Can you work these out from the model? Positions are in its coordinate system, mm. Face numbers are marked on the shaded views. A direction names the side the tool comes from. Round coordinates to 2 decimals unless told otherwise and drop trailing zeros. Write each loop counter-clockwise with the first axis right and the second up, starting at its lowest first coordinate (ties: lowest second). Pieces come first, ordered by that corner, then holes. Notation, with made-up numbers: M 15.25,-19.75 L 21.25,-19.75 A17 ccw 21.25,3.25 Z; hole C -36.75,-15 d7. An arc over 180 degrees is marked long. Answer in a Markdown table with one row per item. Add a question column.
(1) Suppose I cut it at B-B, the plane y = -11. Write out the boundary of the cut face in (x, z), then the cut area to 3 significant figures.
(2) If I drill on probe 1 along X at (y, z) = (-17.65, 0); probe 2 along X at (y, z) = (-14, 0.75); probe 3 along X at (y, z) = (-10, 2.5), over which ranges is the centre line in solid material (lowest first)?
(3) I'm going to push flat-ended pins straight in: pin 1 (2 mm diameter, centred on x = 0, z = 0, fed in from +Y); pin 2 (2 mm diameter, centred on x = 0, z = 0, fed in from -Y); pin 3 (2 mm diameter, centred on x = 1.5, y = 3, fed in from -Z). Where does each tip first touch, or does it pass through?
(4) Suppose I cut it at A-A, the plane y = 17. Write out the boundary of the cut face in (x, z), then the cut area to 3 significant figures.
(5) If we mould it in two halves opening along Z, with no side actions, what happens to the marked faces 1, 2 and 3? For each: released by +Z, released by -Z, zero draft, split by the parting line, or undercut.
(6) For the marked faces 4 and 5, which set-ups out of +Z, -Z, +X, -X, +Y, -Y let a thin tool reach every point of the face, with its end or its side?
Autodesk Inventor part; units mm, degrees
ref_plane "YZ Plane" through (0, 0, 0) normal (1, 0, 0) x (0, 1, 0)
ref_plane "XZ Plane" through (0, 0, 0) normal (0, 1, 0) x (-1, 0, 0)
ref_plane "XY Plane" through (0, 0, 0) normal (0, 0, 1) x (1, 0, 0)
sketch "スケッチ1" plane through (0, 0, 0) normal (1, 0, 0) x (0, 1, 0)
  line L0 (-19.75, 0) -> (19.75, 0)
  line L1 (0, 0) -> (0, 3.4641) construction
  line L2 (-19.4821, 3.4641) -> (-19.75, 3)
  line L3 (-19.75, 3) -> (-19.75, 0)
  line L4 (-19.4821, 3.4641) -> (19.4821, 3.4641)
  line L5 (19.4821, 3.4641) -> (19.75, 3)
  line L6 (19.75, 3) -> (19.75, 0)
  dimension "d1" = 3
  dimension "d2" = 3.4641
  dimension "d3" = 30
  dimension "d4" = 39.5
revolve "回転1" add sketch "スケッチ1" angle 360 about axis through (0, -19.75, 0) along (0, 1, 0)
sketch "スケッチ2" plane through (0, 19.75, 0) normal (0, 1, 0) x (1, 0, 0)
  circle A0 centre (0, 0) radius 3.4641
  line L0 (0, -3.4641) -> (-3, -1.7321)
  line L1 (-3, -1.7321) -> (-3, 1.7321)
  line L2 (-3, 1.7321) -> (0, 3.4641)
  line L3 (0, 3.4641) -> (3, 1.7321)
  line L4 (3, 1.7321) -> (3, -1.7321)
  line L5 (3, -1.7321) -> (0, -3.4641)
  point P0 (0, 0)
  point P1 (0, 0)
  point P2 (3, -1.7321)
  point P3 (3, -1.7321)
  point P4 (3, 1.7321)
  point P5 (3, 1.7321)
  point P6 (0, 3.4641)
  point P7 (0, 3.4641)
  point P8 (-3, 1.7321)
  point P9 (-3, 1.7321)
  point P10 (-3, -1.7321)
  point P11 (-3, -1.7321)
extrude "押し出し1" cut sketch "スケッチ2" against normal through all contours A0 L4 | L3 A0 | A0 L5 | L2 A0 | A0 L0 | L1 A0
hole "穴1" at (0, 19.75, 0) direction (0, -1, 0) diameter 2.459 depth 6 tip angle 118 countersink diameter 3 countersink angle 90
mirror "ミラー1" about plane through (0, 0, 0) normal (0, 1, 0) of "穴1"
equation "\"d2\" = 1.1547 * d1"
properties part number "ABLSBF6-39.5-M3-N3" material "アルミニウム 2014-T4"
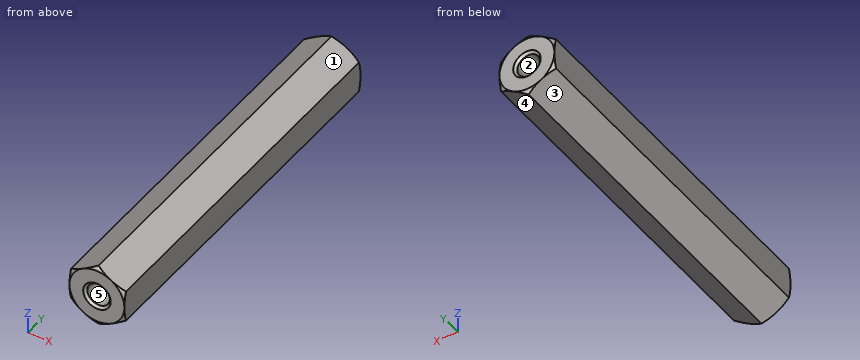
Calculated:
| question | item | result |
|---|---|---|
| 1 | outline | M -3,-1.73 L 0,-3.46 L 3,-1.73 L 3,1.73 L 0,3.46 L -3,1.73 Z |
| 1 | area | 31.2 mm² |
| 2 | probe 1 | -3 to -1.23, 1.23 to 3 |
| 2 | probe 2 | -3 to -0.97, 0.97 to 3 |
| 2 | probe 3 | -1.67 to 1.67 |
| 3 | pin 1 | y = 13.61 |
| 3 | pin 2 | y = -13.61 |
| 3 | pin 3 | z = -3.18 |
| 4 | outline | M -3,-1.73 L 0,-3.46 L 3,-1.73 L 3,1.73 L 0,3.46 L -3,1.73 Z; hole C 0,0 d2.46 |
| 4 | area | 26.4 mm² |
| 5 | face 1 | released by +Z |
| 5 | face 2 | undercut |
| 5 | face 3 | released by -Z |
| 6 | face 4 | -Z, +X, +Y, -Y |
| 6 | face 5 | -Y |
